Geometry check sheet. Reference: the model listing, model coordinates, mm. A direction names the side the tool comes from. Coordinates: 2 decimals unless noted, no trailing zeros. Order: outer loops, then holes, each group sorted by start corner. A loop starts at its lowest first (then second) coordinate and runs counter-clockwise, first axis right, second up. Notation, with made-up numbers: (69, -25) - (91, -25) arc R17 ccw to (91, 7) - close; hole circle Ø6 at (44.5, 87). An arc over 180 degrees is marked (long way). Put each result on its own line as item: value.
Autodesk Inventor part; units mm, degrees
ref_plane "YZ Plane" through (0, 0, 0) normal (1, 0, 0) x (0, 1, 0)
ref_plane "XZ Plane" through (0, 0, 0) normal (0, 1, 0) x (-1, 0, 0)
ref_plane "XY Plane" through (0, 0, 0) normal (0, 0, 1) x (1, 0, 0)
ref_plane "작업 평면1" through (0, 0, 0) normal (0, 0, 1) x (1, 0, 0)
sketch "스케치1" plane through (0, 0, 0) normal (0, 0, 1) x (1, 0, 0)
  circle A0 centre (-7.7782, -7.7782) radius 1.55
  circle A1 centre (7.7782, -7.7782) radius 1.55
  circle A2 centre (7.7782, 7.7782) radius 1.55
  circle A3 centre (-7.7782, 7.7782) radius 1.55
  circle A4 centre (0, 0) radius 5
  circle A5 centre (0, 0) radius 13.9
  circle A6 centre (0, 11) radius 1.55
  circle A7 centre (11, 0) radius 1.55
  circle A8 centre (0, -11) radius 1.55
  circle A9 centre (-11, 0) radius 1.55
  line L0 (-40.1, -17) -> (40.1, -17)
  line L1 (40.1, -17) -> (40.1, 17)
  line L2 (40.1, 17) -> (-40.1, 17)
  line L3 (-40.1, 17) -> (-40.1, -17)
  line L4 (-40.1, -17) -> (40.1, 17) construction
  line L5 (40.1, -17) -> (-40.1, 17) construction
  circle A10 centre (0, 0) radius 7
  circle A11 centre (0, 11) radius 1.35
  circle A12 centre (-7.7782, 7.7782) radius 1.35
  circle A13 centre (-11, 0) radius 1.35
  circle A14 centre (-7.7782, -7.7782) radius 1.35
  circle A15 centre (0, -11) radius 1.35
  circle A16 centre (7.7782, -7.7782) radius 1.35
  circle A17 centre (11, 0) radius 1.35
  circle A18 centre (7.7782, 7.7782) radius 1.35
  line L6 (6, 17) -> (-6, 17)
  line L7 (-6, 17) -> (-6, 23)
  line L8 (-6, 23) -> (6, 23)
  line L9 (6, 23) -> (6, 17)
  line L10 (6, -17) -> (-6, -17)
  line L11 (-6, -17) -> (-6, -23)
  line L12 (-6, -23) -> (6, -23)
  line L13 (6, -23) -> (6, -17)
  point P0 (0, 0)
  point P1 (0, 0)
  point P2 (0, 0)
  point P3 (0, 0)
  point P4 (0, 0)
  point P5 (0, 0)
  point P6 (0, 0)
  point P7 (0, 0)
  dimension "d0" = 80.2
  dimension "d1" = 34
  dimension "d2" = 2
  dimension "d3" = 2.7
  dimension "d6" = 360
  dimension "d8" = 12
  dimension "d9" = 6
  dimension "d10" = 12
  dimension "d11" = 6
extrude "돌출1" add sketch "스케치1" along normal blind 6 contours A5 | L3 L2 L1 L0 | L0 L13 L12 L11 | L7 L8 L9 L2
sketch "스케치3" plane through (-6, 23, 0) normal (0, 1, 0) x (1, 0, 0)
  circle A0 centre (26, -3) radius 1.35
  circle A1 centre (-14, -3) radius 1.35
  point P0 (6, 0)
  dimension "d14" = 2.7
  dimension "d15" = 2.7
extrude "돌출2" cut sketch "스케치3" against normal blind 100
sketch "스케치4" plane through (0, 0, 6) normal (0, 0, 1) x (1, 0, 0)
  line L0 (22.2, 12.7) -> (17, 10.5) construction
  line L1 (17, 12.7) -> (22.2, 10.5) construction
  line L2 (-22.2, 12.7) -> (-17, 10.5) construction
  line L3 (-17, 12.7) -> (-22.2, 10.5) construction
  line L4 (17.8, -12.7) -> (23, -12.7)
  line L5 (23, -10.5) -> (17.8, -10.5)
  line L6 (17.8, -10.5) -> (17.8, -12.7)
  line L7 (17.8, -12.7) -> (23, -10.5) construction
  line L8 (23, -12.7) -> (17.8, -10.5) construction
  line L9 (-22.2, -12.7) -> (-17, -10.5) construction
  line L10 (-17, -12.7) -> (-22.2, -10.5) construction
  line L11 (18.65, 17) -> (18.65, -17)
  line L12 (21.35, 17) -> (21.35, -17)
  line L13 (17.4, 10.5) -> (22.6, 10.5)
  line L14 (22.6, 10.5) -> (22.6, 12.7)
  line L15 (22.6, 12.7) -> (17.4, 12.7)
  line L16 (17.4, 12.7) -> (17.4, 10.5)
  line L17 (17.4, 10.5) -> (22.6, 12.7) construction
  line L18 (22.6, 10.5) -> (17.4, 12.7) construction
  line L19 (-22.6, 10.3308) -> (-17.4, 10.3308)
  line L20 (-17.4, 10.3308) -> (-17.4, 12.5308)
  line L21 (-17.4, 12.5308) -> (-22.6, 12.5308)
  line L22 (-22.6, 12.5308) -> (-22.6, 10.3308)
  line L23 (-22.6, 10.3308) -> (-17.4, 12.5308) construction
  line L24 (-17.4, 10.3308) -> (-22.6, 12.5308) construction
  line L25 (22.6, -12.7) -> (22.6, -10.5)
  line L26 (17.4, -12.7) -> (22.6, -10.5) construction
  line L27 (22.6, -12.7) -> (17.4, -10.5) construction
  line L28 (-22.6, -12.531) -> (-17.4, -12.531)
  line L29 (-17.4, -12.531) -> (-17.4, -10.331)
  line L30 (-17.4, -10.331) -> (-22.6, -10.331)
  line L31 (-22.6, -10.331) -> (-22.6, -12.531)
  line L32 (-22.6, -12.531) -> (-17.4, -10.331) construction
  line L33 (-17.4, -12.531) -> (-22.6, -10.331) construction
  point P0 (0, 0)
  point P1 (-19.6, 11.6)
  point P2 (20.4, -11.6)
  point P3 (-19.6, -11.6)
  point P4 (20, 11.6)
  point P5 (-20, 11.4308)
  point P6 (20, -11.6)
  point P7 (-20, -11.431)
  dimension "d18" = 5.2
  dimension "d19" = 2.2
  dimension "d20" = 5.2
  dimension "d21" = 2.2
  dimension "d22" = 5.2
  dimension "d23" = 2.2
  dimension "d24" = 5.2
  dimension "d25" = 2.2
  dimension "d28" = 5.2
  dimension "d29" = 2.2
  dimension "d30" = 5.2
  dimension "d31" = 2.2
  dimension "d32" = 5.2
  dimension "d33" = 2.2
  dimension "d34" = 5.2
  dimension "d35" = 2.2
extrude "돌출4" cut sketch "스케치4" against normal blind 10 contours L6 L5 L11 L4 | L11 L5 L12 L4 | L12 L5 L25 L4 | L13 L16 L15 L11 | L11 L15 L12 L13 | L12 L15 L14 L13 | L22 L21 L20 L19 | L31 L30 L29 L28
sketch "스케치5" plane through (0, 0, 6) normal (0, 0, 1) x (1, 0, 0)
  line L0 (22.6, 10.5) -> (17.4, 10.5)
  line L1 (17.4, 10.5) -> (17.4, 12.7)
  line L2 (17.4, 12.7) -> (22.6, 12.7)
  line L3 (22.6, 12.7) -> (22.6, 10.5)
  line L4 (-22.6, -10.331) -> (-17.4, -10.331)
  line L5 (-17.4, -10.331) -> (-17.4, -12.531)
  line L6 (-17.4, -12.531) -> (-22.6, -12.531)
  line L7 (-22.6, -12.531) -> (-22.6, -10.331)
  line L8 (17.8, -12.7) -> (17.8, -10.5)
  line L9 (17.8, -10.5) -> (22.6, -10.5)
  line L10 (22.6, -10.5) -> (22.6, -12.7)
  line L11 (22.6, -12.7) -> (17.8, -12.7)
  line L12 (-22.6, 12.5308) -> (-17.4, 12.5308)
  line L13 (-17.4, 12.5308) -> (-17.4, 10.3308)
  line L14 (-17.4, 10.3308) -> (-22.6, 10.3308)
  line L15 (-22.6, 10.3308) -> (-22.6, 12.5308)
  line L16 (40.1, 17) -> (6, 17)
  line L17 (6, 17) -> (6, 23)
  line L18 (6, 23) -> (-6, 23)
  line L19 (-6, 23) -> (-6, 17)
  line L20 (-6, 17) -> (-40.1, 17)
  line L21 (-40.1, 17) -> (-40.1, -17)
  line L22 (-40.1, -17) -> (-6, -17)
  line L23 (-6, -17) -> (-6, -23)
  line L24 (-6, -23) -> (6, -23)
  line L25 (6, -23) -> (6, -17)
  line L26 (6, -17) -> (40.1, -17)
  line L27 (40.1, -17) -> (40.1, 17)
  circle A0 centre (-7.7782, -7.7782) radius 1.55
  circle A1 centre (7.7782, -7.7782) radius 1.55
  circle A2 centre (7.7782, 7.7782) radius 1.55
  circle A3 centre (-7.7782, 7.7782) radius 1.55
  circle A4 centre (0, 11) radius 1.55
  circle A5 centre (11, 0) radius 1.55
  circle A6 centre (0, -11) radius 1.55
  circle A7 centre (-11, 0) radius 1.55
  circle A8 centre (0, 0) radius 7
  circle A9 centre (6, 17) radius 1
  circle A10 centre (-6, 17) radius 1
  circle A11 centre (6, -17) radius 1
  circle A12 centre (-6, -17) radius 1
  point P0 (0, 0)
  point P1 (-6, 18)
  point P2 (-7, 17)
  point P3 (6, 18)
  point P4 (7, 17)
  point P5 (7, -17)
  point P6 (6, -18)
  dimension "d38" = 2
  dimension "d39" = 2
  dimension "d40" = 2
  dimension "d41" = 2
extrude "돌출5" cut sketch "스케치5" against normal blind 10 contours A9 L17 L16 | L26 L25 A11 | A10 L20 L19 | A12 L22 L23 | L23 L22 A12 picked at (6.5384, 16.6156) picked at (6.5384, -16.6156) picked at (-6.657, 16.9202)
properties part number "hip joint_body connector" material "PMMA 플라스틱"
Q1. Section check D-D on x = 0. Record the boundary of the cut face in (y, z).
Answer block:
outline: (-23, 0) - (-12.55, 0) - (-12.55, 6) - (-23, 6) - close; (-9.45, 0) - (-7, 0) - (-7, 6) - (-9.45, 6) - close; (7, 0) - (9.45, 0) - (9.45, 6) - (7, 6) - close; (12.55, 0) - (23, 0) - (23, 6) - (12.55, 6) - close
Q2. Depth check by flat-ended pin: pin 1 Ø3.5 at (x, z) = (-20, 3) entering from -Y. Enter the tip coordinate at first touch or a pass-through.
Answer block:
pin 1: stops at y = -17
Q3. Section check B-B on x = 11. Record the boundary of the cut face in (y, z), then the cut area to 3 significant figures.
Answer block:
outline: (-17, 0) - (-1.55, 0) - (-1.55, 6) - (-17, 6) - close; (1.55, 0) - (17, 0) - (17, 6) - (1.55, 6) - close
area: 185 mm^2
Q4. Thickness scan on L1, parallel to Y at x = -22, z = 4.9; L2, parallel to X at y = 13.5, z = 3.8; L3, parallel to X at y = -13.5, z = 3.1. Record the ranges inside material, lowest first. Write a range as [from, to].
Answer block:
L1: y = [-17, -12.53], [-10.33, 10.33], [12.53, 17]
L2: x = [-40.1, -21.09], [-18.91, 18.91], [21.09, 40.1]
L3: x = [-40.1, -21.35], [-18.65, 18.65], [21.35, 40.1]
Q5. Access from +Z, -Z, +X, -X, +Y, -Y to the whole of each face (thin tool, end or side, straight path). Record for faces 1 (the flat face through (-6, 20, 3)), 2 (the flat face through (-40.1, 0, 3)), 3 (the flat face through (-22.6, -11, 3)).
Answer block:
face 1: +Z, -Z, -X, +Y
face 2: +Z, -Z, -X, +Y, -Y
face 3: +Z, -Z
Q6. Draft check along X on faces 4 (the flat face through (17.4, 12, 3)), 5 (the flat face through (-6, -20, 3)), 6 (the flat face through (-23, 17, 3)), 7 (the cylindrical face through (-18.712, -14.734, 2.594)). Enter one of: pulls with the +X half, pulls with the -X half, needs draft (parallel to the pull), parting line crosses it, or undercut.
Answer block:
face 4: undercut
face 5: pulls with the -X half
face 6: needs draft
face 7: undercut
Q7. Section check A-A on y = 0. Record the boundary of the cut face in (x, z), then the cut area to 3 significant figures.
Answer block:
outline: (-40.1, 0) - (-12.55, 0) - (-12.55, 6) - (-40.1, 6) - close; (-9.45, 0) - (-7, 0) - (-7, 6) - (-9.45, 6) - close; (7, 0) - (9.45, 0) - (9.45, 6) - (7, 6) - close; (12.55, 0) - (40.1, 0) - (40.1, 6) - (12.55, 6) - close; hole circle Ø2.7 at (-20, 3); hole circle Ø2.7 at (20, 3)
area: 349 mm^2
Q8. Section check C-C on x = 20. Record the boundary of the cut face in (y, z).
Answer block:
outline: (-17, 0) - (-12.7, 0) - (-12.7, 1.65) - (-17, 1.65) - close; (-17, 4.35) - (-12.7, 4.35) - (-12.7, 6) - (-17, 6) - close; (-10.5, 0) - (10.5, 0) - (10.5, 1.65) - (-10.5, 1.65) - close; (-10.5, 4.35) - (10.5, 4.35) - (10.5, 6) - (-10.5, 6) - close; (12.7, 0) - (17, 0) - (17, 1.65) - (12.7, 1.65) - close; (12.7, 4.35) - (17, 4.35) - (17, 6) - (12.7, 6) - close
